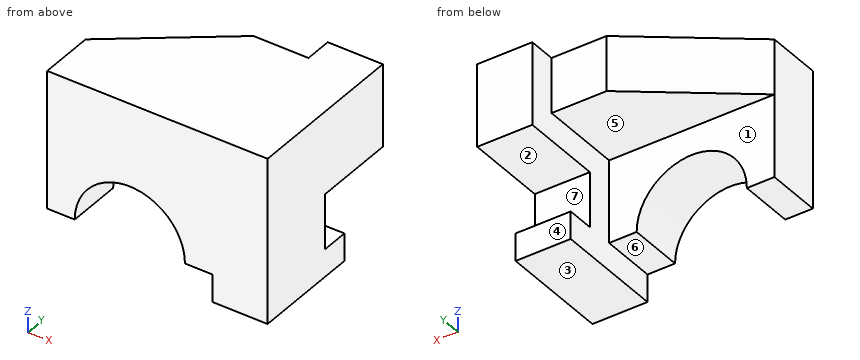
from build123d import *

# Parameters (mm, degrees)
SALIENTE_EXTRUIR1_DEPTH = 200
CROQUIS3_W              = 600
CROQUIS3_H              = 200
SALIENTE_EXTRUIR2_DEPTH = 600
CORTAR_EXTRUIR1_REACH   = 783.025
CROQUIS4_W              = 600
CROQUIS4_H              = 100
CORTAR_EXTRUIR2_REACH   = 783.025
CROQUIS6_W              = 600
CROQUIS6_H              = 200
SALIENTE_EXTRUIR3_DEPTH = 300
CORTAR_EXTRUIR3_DEPTH   = 200


with BuildPart() as part:
    # Croquis2 → Saliente-Extruir1 (new body)
    with BuildSketch(Plane(origin=(0, 0, 0), x_dir=(0, 0, -1), z_dir=(1, 0, 0))):
        Polygon((-300, -300), (300, -300), (300, 0), (300, 100), (200, 100), (200, 0), (0, 0), (0, 300), (-300, 300), align=None)
    extrude(amount=SALIENTE_EXTRUIR1_DEPTH)

    # Croquis3 → Saliente-Extruir2 (add)
    with BuildSketch(Plane.ZY):
        with Locations((0, -200)):
            Rectangle(CROQUIS3_W, CROQUIS3_H)
    extrude(amount=SALIENTE_EXTRUIR2_DEPTH)

    # Croquis4 → Cortar-Extruir1 (cut, up to next)
    with BuildSketch(Plane(origin=(0, -100, 0), x_dir=(1, 0, 0), z_dir=(0, 1, 0)), mode=Mode.PRIVATE) as cortar_extruir1_sk1:
        with Locations((-300, 250)):
            Rectangle(CROQUIS4_W, CROQUIS4_H)
    cortar_extruir1_tool1 = extrude(cortar_extruir1_sk1.sketch, amount=-CORTAR_EXTRUIR1_REACH, mode=Mode.PRIVATE) & part.part
    add(cortar_extruir1_tool1.solids().sort_by_distance((-300, -100, -250))[0], mode=Mode.SUBTRACT)

    # Croquis5 → Cortar-Extruir2 (cut, up to next)
    with BuildSketch(Plane(origin=(0, -100, 0), x_dir=(1, 0, 0), z_dir=(0, 1, 0)), mode=Mode.PRIVATE) as cortar_extruir2_sk1:
        with BuildLine():
            Line((-500, 200), (-100, 200))
            ThreePointArc((-100, 200), (-300, 0), (-500, 200))
        make_face()
    cortar_extruir2_tool1 = extrude(cortar_extruir2_sk1.sketch, amount=-CORTAR_EXTRUIR2_REACH, mode=Mode.PRIVATE) & part.part
    add(cortar_extruir2_tool1.solids().sort_by_distance((-300, -100, -115.117364))[0], mode=Mode.SUBTRACT)

    # Croquis6 → Saliente-Extruir3 (add)
    with BuildSketch(Plane(origin=(0, -100, 0), x_dir=(1, 0, 0), z_dir=(0, 1, 0))):
        with Locations((-300, -200)):
            Rectangle(CROQUIS6_W, CROQUIS6_H)
    extrude(amount=SALIENTE_EXTRUIR3_DEPTH)

    # Croquis7 → Cortar-Extruir3 (cut)
    with BuildSketch(Plane(origin=(0, 0, 100), x_dir=(-1, 0, 0), z_dir=(0, 0, -1))):
        Polygon((200, 200), (600, -100), (600, 200), align=None)
    extrude(amount=-CORTAR_EXTRUIR3_DEPTH, mode=Mode.SUBTRACT)


solid = part.part
Check sheet for the modelled part. Datum: model origin and axes. Units: mm. Face numbers are marked on the shaded views. A direction names the side the tool comes from. Coordinates: 2 decimals unless noted, no trailing zeros. Write each loop counter-clockwise with the first axis right and the second up, starting at its lowest first coordinate (ties: lowest second). Pieces come first, ordered by that corner, then holes. Notation, with made-up numbers: M -35,81 L 17,81 A19 ccw 17,104 Z; hole C 89.5,-7.5 d2. An arc over 180 degrees is marked long. Answer as CSV lines item,"result".
Q1. Material ranges on probe 1 along X at (y, z) = (260.5, 222); probe 2 along Y at (x, z) = (-352, 69); probe 3 along Z at (x, y) = (-322, -10.5), recorded low to high. Write a range as from..to.
Check result:
probe 1,"0..200"
probe 2,"-300..-100"
probe 3,"100..300"
Q2. Mould release check, pull along Z, two halves, no side actions. Record for the marked faces 1, 2 and 3: released by +Z, released by -Z, zero draft, split by the parting line, or undercut.
Check result:
face 1,"zero draft"
face 2,"undercut"
face 3,"released by -Z"
Q3. Cross-section at B-B (z = -138). Record the boundary of the cut face in (x, y), then the cut area to 3 significant figures.
Check result:
outline,"M -600,-300 L -490.15,-300 L -490.15,-100 L -600,-100 Z; M -109.85,-300 L 200,-300 L 200,0 L 0,0 L 0,-100 L -109.85,-100 Z"
area,"104,000 mm^2"
Q4. Cross-section at D-D (y = -111). Record the boundary of the cut face in (x, z).
Check result:
outline,"M -600,-200 L -500,-200 A200 cw -100,-200 L 0,-200 L 0,-300 L 200,-300 L 200,300 L -600,300 Z"
Q5. Cross-section at C-C (z = 153.5). Record the boundary of the cut face in (x, y), then the cut area to 3 significant figures.
Check result:
outline,"M -600,-300 L 200,-300 L 200,300 L 0,300 L 0,200 L -200,200 L -600,-100 Z"
area,"360,000 mm^2"
Q6. Go/stop test with flat-tipped pins: pin 1 (8 mm diameter, centred on x = -7.5, y = 3, fed in from -Z); pin 2 (6 mm diameter, centred on x = -107.5, z = -113.5, fed in from +Y). Record where each tip stops, or that it passes through.
Check result:
pin 1,"z = 100"
pin 2,"y = -100"
Q7. Set-up check for the marked faces 4, 5, 6 and 7: record each of +Z, -Z, +X, -X, +Y, -Y from which the full face is reachable in a straight line by a thin tool's end or side.
Check result:
face 4,"-Z, +X, -X, +Y"
face 5,"-Z, -X, +Y"
face 6,"-Z, -X, +Y, -Y"
face 7,"+X, -X, +Y"
Q8. Cross-section at A-A (y = 15.5). Record the boundary of the cut face in (x, z), then the cut area to 3 significant figures.
Check result:
outline,"M -446,100 L 0,100 L 0,0 L 200,0 L 200,300 L -446,300 Z; M 0,-300 L 200,-300 L 200,-200 L 0,-200 Z"
area,"169,000 mm^2"
